Here's the drawing with two shaded views (mm, measured from the low corner). I have some questions. Coordinates: 2 decimals unless noted, no trailing zeros. Write each loop counter-clockwise with the first axis right and the second up, starting at its lowest first coordinate (ties: lowest second). Pieces come first, ordered by that corner, then holes.
Item 1: I want a section at B-B on z = 2. Please give me the cut outline in (x, y), then the cut area to 3 significant figures.
Item 2: I want a section at C-C on x = 10.25. Please give me the cut outline in (y, z).
Item 3: I want a section at D-D on x = 13.7. State how many separate pieces and enclosed holes the cut face has, then the cut area to 3 significant figures.
Item 4: I want a section at A-A on x = 2.7. Please give me the cut outline in (y, z).
Item 5: For P1, Ø8, axis at x = 12.5, z = 3.5, coming from the -Y side; P2, Ø2, axis at x = 11.43, z = 13.59, coming from the +Y side; P3, Ø0.5, axis at y = 1.5, z = 9.5, coming from the +X side; P4, Ø0.8, axis at y = 1.5, z = 8, coming from the -X side, each with a flat end and sliding along its axis, tell me the tip position at first contact or that it passes through.
Item 6: If I drill on probe 1 along X at (y, z) = (0.25, 2); probe 2 along X at (y, z) = (0.2, 1); probe 3 along Z at (x, y) = (12, 1.3), over which ranges is the centre line in solid material (lowest first)?
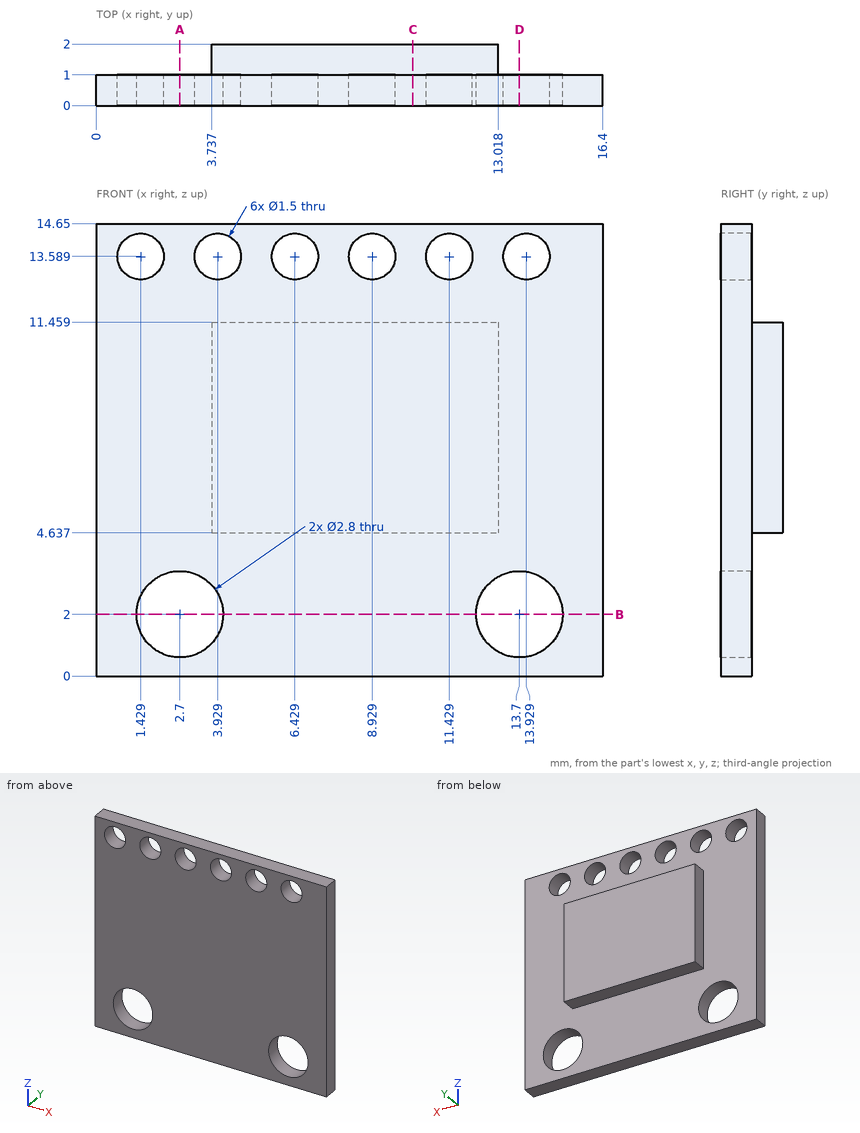
Response values:
1. outline: (0, 0) - (1.3, 0) - (1.3, 1) - (0, 1) - close; (4.1, 0) - (12.3, 0) - (12.3, 1) - (4.1, 1) - close; (15.1, 0) - (16.4, 0) - (16.4, 1) - (15.1, 1) - close
1. area: 10.8 mm2
2. outline: (0, 0) - (1, 0) - (1, 4.64) - (2, 4.64) - (2, 11.46) - (1, 11.46) - (1, 14.65) - (0, 14.65) - close
3. separate pieces: 3
3. enclosed holes: 0
3. area: 10.4 mm2
4. outline: (0, 0) - (1, 0) - (1, 0.6) - (0, 0.6) - close; (0, 3.4) - (1, 3.4) - (1, 14.65) - (0, 14.65) - close
5. P1: stops at y = 0
5. P2: stops at y = 1
5. P3: stops at x = 13.02
5. P4: stops at x = 3.74
6. probe 1: x = 0 to 1.3, 4.1 to 12.3, 15.1 to 16.4
6. probe 2: x = 0 to 1.72, 3.68 to 12.72, 14.68 to 16.4
6. probe 3: z = 4.64 to 11.46
